```python
from build123d import *

# Parameters (mm, degrees)
F1_DEPTH = 80
F3_DEPTH = 36
F4_R     = 20
F5_R     = 5
F6_R     = 39.99999
F8_DEPTH = 85


# Not quite as in the source:
# - a fillet or chamfer is up to 0.001 mm smaller than in the source, because OpenCascade refuses the exact size


with BuildPart() as f1:
    # F0 (on Top) → F1 (new body)
    with BuildSketch(Plane.XY):
        Polygon((-40, 69.2820323028), (0, 0), (150, 0), (150, 10), (40.4145188433, 10), (-5.3589838486, 89.2820323028), (-14.0192378865, 84.2820323028), (15.9807621135, 32.3205080757), (-1.3397459622, 22.3205080757), (-31.3397459622, 74.2820323028), align=None)
    extrude(amount=F1_DEPTH)

    # F2 (on face) → F3 (cut)
    with BuildSketch(Plane(origin=(0, 10, 0), x_dir=(-1, 0, 0), z_dir=(0, 1, 0))):
        with BuildLine():
            Line((-90, 40), (-150, 40))
            Line((-150, 40), (-150, 30))
            Line((-150, 30), (-100, 30))
            ThreePointArc((-100, 30), (-92.9289321881, 32.9289321881), (-90, 40))
        make_face()
        with BuildLine():
            Line((-150, 50), (-150, 40))
            Line((-150, 40), (-90, 40))
            ThreePointArc((-90, 40), (-92.9289321881, 47.0710678119), (-100, 50))
            Line((-100, 50), (-150, 50))
        make_face()
    extrude(amount=-F3_DEPTH, mode=Mode.SUBTRACT)

    # F4
    f4_edges = [f1.edges().sort_by_distance(p)[0] for p in [
        (150, 5, 80),
        (150, 5, 0),
    ]]
    fillet(f4_edges, radius=F4_R)

    # F5
    f5_edges = [f1.edges().sort_by_distance(p)[0] for p in [
        (40.414519, 10, 40),
    ]]
    fillet(f5_edges, radius=F5_R)

    # F6 (radius 40 in the source; OpenCascade refuses exactly that, so slightly less here)
    f6_edges = [f1.edges().sort_by_distance(p)[0] for p in [
        (-9.689111, 86.782032, 0),
        (-35.669873, 71.782032, 0),
        (-9.689111, 86.782032, 80),
        (-35.669873, 71.782032, 80),
    ]]
    fillet(f6_edges, radius=F6_R)

    # F7 (on face) → F8 (cut)
    with BuildSketch(Plane(origin=(34.6410161514, 20, 0), x_dir=(-0.5, 0.8660254038, 0), z_dir=(0.8660254038, 0.5, 0))):
        with BuildLine():
            ThreePointArc((50.0682017207, 40), (47.1151153286, 47.0951397875), (40, 49.9997674236))
            ThreePointArc((40, 49.9997674236), (32.9730619333, 47.0469136078), (30.0682017207, 40))
            ThreePointArc((30.0682017207, 40), (32.9730619333, 32.9530863922), (40, 30.0002325764))
            ThreePointArc((40, 30.0002325764), (47.1151153286, 32.9048602125), (50.0682017207, 40))
        make_face()
    extrude(amount=-F8_DEPTH, mode=Mode.SUBTRACT)


solid = f1.part
```
Design review of the part built by this model. Coordinates are the model's own, in mm. A direction names the side the tool comes from. Give positions to 0.01 mm unless a question says otherwise; leave off trailing zeros. Write each loop counter-clockwise with the first axis right and the second up, starting at its lowest first coordinate (ties: lowest second). Pieces come first, ordered by that corner, then holes.
(1) Wall thickness on line 1 along X through (y, z) = (67.5, 39.5); line 2 along Y through (x, z) = (58, 29); line 3 along X through (y, z) = (42.5, 20): over which ranges is each line inside the solid? List them lowest first.
Checked values:
line 1: x = -38.97 to -27.42, -4.33 to 7.22
line 2: y = 0 to 10
line 3: x = -24.54 to -12.99, 10.1 to 21.65
(2) Add section D-D (z = 35). Give the boundary of the cut face in (x, y).
Checked values:
outline: (-39.84, 69.01) - (-24.36, 42.2) - (-15.7, 47.2) - (-31.18, 74.01) - close; (-15.7, 27.2) - (0, 0) - (91.34, 0) - (91.34, 10) - (43.3, 10) arc R5 cw to (38.97, 12.5) - (18.94, 47.2) - (10.28, 42.2) - (15.98, 32.32) - (-1.34, 22.32) - (-7.04, 32.2) - close; (-13.86, 84.01) - (1.62, 57.2) - (10.28, 62.2) - (-5.2, 89.01) - close
(3) Clearance check with flat-ended pins moving along their axes: pin 1 Ø10 at (y, z) = (55, 11.5) entering from +X; pin 2 Ø6 at (y, z) = (43.5, 35.5) entering from +X; pin 3 Ø2 at (y, z) = (35, 28.5) entering from +X. State where each tip first meets the part, or that it passes through.
Checked values:
pin 1: stops at x = 17.32
pin 2: stops at x = 22.81
pin 3: stops at x = 26.56
(4) Add section C-C (z = 22). Give the boundary of the cut face in (x, y).
Checked values:
outline: (-37.86, 65.58) - (0, 0) - (150, 0) - (150, 10) - (43.3, 10) arc R5 cw to (38.97, 12.5) - (-3.22, 85.58) - (-11.88, 80.58) - (15.98, 32.32) - (-1.34, 22.32) - (-29.2, 70.58) - close
(5) Add section B-B (x = 49). Give the boundary of the cut face in (y, z), and give its area (3 significant figures).
Checked values:
outline: (0, 0) - (10, 0) - (10, 80) - (0, 80) - close
area: 800 mm2
(6) Tool access review of faces 5 (the face through (-29.72, 61.33, 11.41)), 6 (the face through (38, 11, 0)), 7 (the face through (0.77, 58.67, 39.44)), 8 (the face through (86, 10, 39)), 9 (the face through (125, 5, 30)): name each direction out of +Z, -Z, +X, -X, +Y, -Y from which nothing blocks a thin tool from reaching the whole face with its end or side.
Checked values:
face 5: -Z, -X, +Y
face 6: -Z, +X, -X, +Y, -Y
face 7: +Z, -Z
face 8: +Z, -Z, +X, +Y
face 9: +X, +Y, -Y
(7) Add section A-A (z = 44). Give the boundary of the cut face in (x, y).
Checked values:
outline: (-39.9, 69.11) - (-24.62, 42.64) - (-15.96, 47.64) - (-31.24, 74.11) - close; (-15.45, 26.76) - (0, 0) - (90.83, 0) - (90.83, 10) - (43.3, 10) arc R5 cw to (38.97, 12.5) - (19.19, 46.76) - (10.53, 41.76) - (15.98, 32.32) - (-1.34, 22.32) - (-6.79, 31.76) - close; (-13.92, 84.11) - (1.36, 57.64) - (10.02, 62.64) - (-5.26, 89.11) - close
(8) Mouldability with a two-part tool opening along X and no side actions: class faces 1 (the face through (125, 5, 50)), 2 (the face through (-3.74, 76.33, 11.41)), 3 (the face through (7.44, 27.39, 39.44)), 4 (the face through (40.833, 10.652, 40.56)) as +X half, -X half, draft (parallel to the pull), parting line (faces both ways), or undercut.
Checked values:
face 1: draft
face 2: -X half
face 3: undercut
face 4: +X half
